Build history of the part. All positions in model axes, mm. Face numbers are marked on the shaded views. A direction names the side the tool comes from. Round coordinates to 2 decimals unless told otherwise and drop trailing zeros. Order: outer loops, then holes, each group sorted by start corner. A loop starts at its lowest first (then second) coordinate and runs counter-clockwise, first axis right, second up. Notation, with made-up numbers: (7.5, -27) -> (12.5, -27) arc R28 cw to (12.5, 2) -> close; hole circle Ø5 at (17, -6). An arc over 180 degrees is marked (long way). Answer as CSV lines item,"result". Start each with the question number.
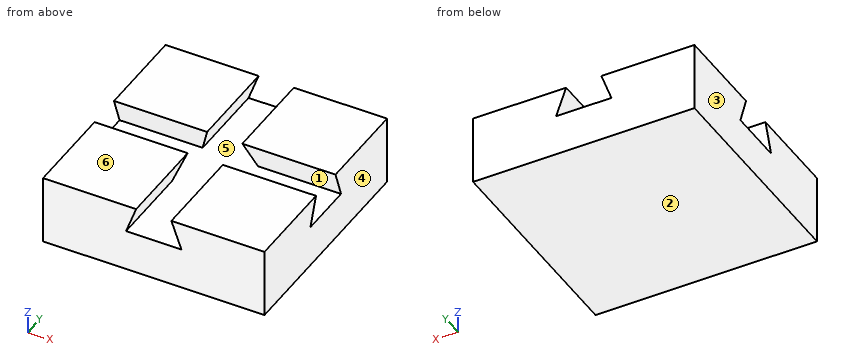
```python
from build123d import *

# Parameters (mm, degrees)
F1_DEPTH = 80
F3_DEPTH = 80


with BuildPart() as f1:
    # F0 (on Front) → F1 (new body)
    with BuildSketch(Plane.XZ):
        Polygon((37.330411, -5.82836), (3.690411, -5.82836), (7.330411, -15.82836), (-12.669589, -15.82836), (-9.029589, -5.82836), (-42.669589, -5.82836), (-42.669589, -30.82836), (37.330411, -30.82836), align=None)
    extrude(amount=-F1_DEPTH)

    # F2 (on face) → F3 (cut)
    with BuildSketch(Plane.YZ.offset(37.330411)):
        Polygon((30, -15.82836), (50, -15.82836), (46.36, -5.82836), (40, -5.82836), (33.64, -5.82836), align=None)
    extrude(amount=-F3_DEPTH, mode=Mode.SUBTRACT)


solid = f1.part
```
Q1. Slice it at B-B, the plane y = 14.5. Write the cut outline in (x, z), plus the area to 3 significant figures.
Q2. Two-plate mould, pull along X, no slides. Class the marked faces 3, 4, 5 and 6: +X half, -X half, draft (parallel to the pull), parting line (faces both ways), or undercut.
Q3. Slice it at A-A, the plane x = -10. Write the cut outline in (y, z).
Q4. Slice it at C-C, the plane x = -27.5. Write the cut outline in (y, z).
Q5. Slice it at D-D, the plane y = 48.5. Write the cut outline in (x, z).
Q6. Probe L1, parallel to Z at x = -31.5, y = 40; L2, parallel to Y at x = -25, z = -8; L3, parallel to X at y = 22, z = -10.75. List the from-to ranges inside material, lowest first.
Q7. Which spindle directions (+Z, -Z, +X, -X, +Y, -Y) get a long thin tool onto all of the face, cutting with end or side? Do the marked faces 1 and 2. Say none if no direction does.
Solutions:
1,outline,"(-42.67, -30.83) -> (37.33, -30.83) -> (37.33, -5.83) -> (3.69, -5.83) -> (7.33, -15.83) -> (-12.67, -15.83) -> (-9.03, -5.83) -> (-42.67, -5.83) -> close"
1,area,"1,840 mm2"
2,face 3,"-X half"
2,face 4,"+X half"
2,face 5,"undercut"
2,face 6,"draft"
3,outline,"(0, -30.83) -> (80, -30.83) -> (80, -15.83) -> (0, -15.83) -> close; (0, -8.49) -> (32.67, -8.49) -> (33.64, -5.83) -> (0, -5.83) -> close; (46.36, -5.83) -> (47.33, -8.49) -> (80, -8.49) -> (80, -5.83) -> close"
4,outline,"(0, -30.83) -> (80, -30.83) -> (80, -5.83) -> (46.36, -5.83) -> (50, -15.83) -> (30, -15.83) -> (33.64, -5.83) -> (0, -5.83) -> close"
5,outline,"(-42.67, -30.83) -> (37.33, -30.83) -> (37.33, -15.83) -> (-42.67, -15.83) -> close; (-42.67, -11.71) -> (-11.17, -11.71) -> (-9.03, -5.83) -> (-42.67, -5.83) -> close; (3.69, -5.83) -> (5.83, -11.71) -> (37.33, -11.71) -> (37.33, -5.83) -> close"
6,L1,"z = -30.83 to -15.83"
6,L2,"y = 0 to 32.85, 47.15 to 80"
6,L3,"x = -42.67 to -10.82, 5.48 to 37.33"
7,face 1,"+X, -X"
7,face 2,"-Z, +X, -X, +Y, -Y"
